```python
from build123d import *

# Parameters (mm, degrees)
SKETCH1_R           = 20
SKETCH1_W           = 5
SKETCH1_H           = 5
BOSS_EXTRUDE1_DEPTH = 5


with BuildPart() as part:
    # Sketch1 → Boss-Extrude1 (new body)
    with BuildSketch(Plane.XY):
        Circle(SKETCH1_R)
        Polygon((12.701705922, 0), (6.350852961, 11), (-6.350852961, 11), (-12.701705922, 0), (-6.350852961, -11), (6.350852961, -11), align=None, mode=Mode.SUBTRACT)
        with Locations((0, 15.5)):
            Rectangle(SKETCH1_W, SKETCH1_H, mode=Mode.SUBTRACT)
        Polygon((16.838457268, 6.834936491), (12.508330249, 4.334936491), (10.008330249, 8.665063509), (14.338457268, 11.165063509), align=None, mode=Mode.SUBTRACT)
        Polygon((14.338457268, -11.165063509), (10.008330249, -8.665063509), (12.508330249, -4.334936491), (16.838457268, -6.834936491), align=None, mode=Mode.SUBTRACT)
        with Locations((0, -15.5)):
            Rectangle(SKETCH1_W, SKETCH1_H, mode=Mode.SUBTRACT)
        Polygon((-16.838457268, -6.834936491), (-12.508330249, -4.334936491), (-10.008330249, -8.665063509), (-14.338457268, -11.165063509), align=None, mode=Mode.SUBTRACT)
        Polygon((-14.338457268, 11.165063509), (-10.008330249, 8.665063509), (-12.508330249, 4.334936491), (-16.838457268, 6.834936491), align=None, mode=Mode.SUBTRACT)
    extrude(amount=BOSS_EXTRUDE1_DEPTH)


solid = part.part
```
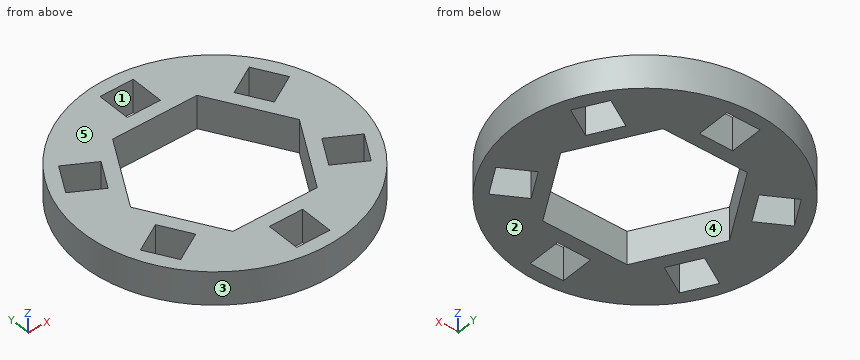
Model file for the job. Use its own axes, mm. Face numbers are marked on the shaded views. A direction names the side the tool comes from. Coordinates: 2 decimals unless noted, no trailing zeros. Order: outer loops, then holes, each group sorted by start corner. A loop starts at its lowest first (then second) coordinate and runs counter-clockwise, first axis right, second up. Notation, with made-up numbers: (19.25, -24) - (28.25, -24) arc R19 ccw to (28.25, -5) - close; hole circle Ø10 at (25, 20). An arc over 180 degrees is marked (long way). Return JSON: item names as keys, results as strings. Group by question number.
1) Saw through at C-C, the plane y = -2. Write the cut outline in (x, z).
2) Saw through at B-B, the plane x = 0. Write the cut outline in (y, z).
3) Tool access for the marked faces 4 and 5: list every direction of +Z, -Z, +X, -X, +Y, -Y with a clear straight run to the whole face (end or side of a thin tool).
4) Saw through at D-D, the plane y = 6. Write the cut outline in (x, z), plus the area to 3 significant figures.
5) Flat gauge pins, fed straight in: P1, Ø3, axis at x = -7.5, z = 3.5, coming from the -Y side; P2, Ø1.5, axis at x = 2.5, z = 3.5, coming from the +Y side; P3, Ø1, axis at y = 5.5, z = 4, coming from the -X side. Where does each tip first touch, or does it go through?
6) Probe line 1 (Y direction, x = -11, z = 1.2); line 2 (X direction, y = -8, z = 0.85); line 3 (Y direction, x = -15.5, z = 2.75). List the from-to ranges inside material, lowest first. Write a range as from..to.
7) Saw through at A-A, the plane z = 2.6. Count the separate pieces of the cut face and the enclosed holes in it, plus the area to 3 significant figures.
8) Mould opens along X. For the marked faces 1, 2 and 3 say: released by +X, released by -X, zero draft, split by the parting line, or undercut.
Values found:
{
 "1": {"outline": "(-19.9, 0) - (-11.55, 0) - (-11.55, 5) - (-19.9, 5) - close; (11.55, 0) - (19.9, 0) - (19.9, 5) - (11.55, 5) - close"},
 "2": {"outline": "(-20, 0) - (-18, 0) - (-18, 5) - (-20, 5) - close; (-13, 0) - (-11, 0) - (-11, 5) - (-13, 5) - close; (11, 0) - (13, 0) - (13, 5) - (11, 5) - close; (18, 0) - (20, 0) - (20, 5) - (18, 5) - close"},
 "3": {"face 4": "+Z, -Z", "face 5": "+Z, +X, -X, +Y, -Y"},
 "4": {"outline": "(-19.08, 0) - (-15.39, 0) - (-15.39, 5) - (-19.08, 5) - close; (-11.55, 0) - (-9.24, 0) - (-9.24, 5) - (-11.55, 5) - close; (9.24, 0) - (11.55, 0) - (11.55, 5) - (9.24, 5) - close; (15.39, 0) - (19.08, 0) - (19.08, 5) - (15.39, 5) - close", "area": "60.0 mm²"},
 "5": {"P1": "stops at y = -19.08", "P2": "stops at y = 19.92", "P3": "stops at x = -19.36"},
 "6": {"line 1": "y = -16.7..-9.24, -6.95..-2.95, 2.95..6.95, 9.24..16.7", "line 2": "x = -18.33..-16.17, -10.39..-8.08, 8.08..10.39, 16.17..18.33", "line 3": "y = -12.64..-9.15, -6.06..6.06, 9.15..12.64"},
 "7": {"separate pieces": "1", "enclosed holes": "7", "area": "687 mm²"},
 "8": {"face 1": "undercut", "face 2": "zero draft", "face 3": "split by the parting line"}
}
